Build history of the part. All positions in model axes, mm. Give positions to 0.01 mm unless a question says otherwise; leave off trailing zeros. Loops run counter-clockwise (first coordinate to the right, second up) from the corner with the lowest first, then second, coordinate; pieces in that order, holes last. Notation, with made-up numbers: (82.5, 31.25) -> (116.5, 31.25) arc R35 ccw to (116.5, 64.25) -> close; hole circle Ø3 at (46, 68). An arc over 180 degrees is marked (long way). Answer as a JSON object with one key per item and string values. Group by question number.
from build123d import *

# Parameters (mm, degrees)
SKETCH1_W           = 12.7
SKETCH1_H           = 20.32
BOSS_EXTRUDE1_DEPTH = 1
SKETCH2_R           = 0.5
SKETCH2_R_2         = 1.0922
CUT_EXTRUDE2_DEPTH  = 1
SKETCH3_W           = 0.7
SKETCH3_H           = 1.6
SKETCH3_W_2         = 2.149156966
SKETCH3_H_2         = 1.228089695
SKETCH3_W_3         = 4.14480272
SKETCH3_H_3         = 2.763201813
SKETCH3_W_4         = 0.8
SKETCH3_H_4         = 1.8
SKETCH3_W_5         = 1.6
SKETCH3_H_5         = 0.7
BOSS_EXTRUDE3_DEPTH = 0.75


with BuildPart() as part:
    # Sketch1 → Boss-Extrude1 (new body)
    with BuildSketch(Plane(origin=(0, 0, 0), x_dir=(1, 0, 0), z_dir=(0, 1, 0))):
        with Locations((6.35, 10.16)):
            Rectangle(SKETCH1_W, SKETCH1_H)
    extrude(amount=BOSS_EXTRUDE1_DEPTH)

    # Sketch2 → Cut-Extrude2 (cut)
    with BuildSketch(Plane(origin=(0, 1, 0), x_dir=(1, 0, 0), z_dir=(0, 1, 0))):
        with Locations(Location((1, 19.32, 0), (0, 0, 270))):
            Circle(SKETCH2_R)
        with Locations(Location((1, 16.702857143, 0), (0, 0, 270))):
            Circle(SKETCH2_R)
        with Locations(Location((1, 14.085714286, 0), (0, 0, 270))):
            Circle(SKETCH2_R)
        with Locations(Location((1, 11.468571429, 0), (0, 0, 270))):
            Circle(SKETCH2_R)
        with Locations(Location((1, 8.851428571, 0), (0, 0, 270))):
            Circle(SKETCH2_R)
        with Locations(Location((1, 6.234285714, 0), (0, 0, 270))):
            Circle(SKETCH2_R)
        with Locations(Location((1, 3.617142857, 0), (0, 0, 270))):
            Circle(SKETCH2_R)
        with Locations(Location((1, 1, 0), (0, 0, 270))):
            Circle(SKETCH2_R)
        with Locations(Location((10.7, 2, 0), (0, 0, 270))):
            Circle(SKETCH2_R_2)
    extrude(amount=-CUT_EXTRUDE2_DEPTH, mode=Mode.SUBTRACT)

    # Sketch3 → Boss-Extrude3 (add)
    with BuildSketch(Plane(origin=(0, 1, 0), x_dir=(1, 0, 0), z_dir=(0, 1, 0))):
        with Locations((9.600163685, 18.251782562)):
            Rectangle(SKETCH3_W, SKETCH3_H)
        with Locations((4.072917024, 18.06582741)):
            Rectangle(SKETCH3_W_2, SKETCH3_H_2)
        with Locations((8.908520197, 9.929733183)):
            Rectangle(SKETCH3_W_3, SKETCH3_H_3)
        with Locations((4.882280256, 4.84279592)):
            Rectangle(SKETCH3_W_4, SKETCH3_H_4)
        with Locations((4.472917024, 2.130764511)):
            Rectangle(SKETCH3_W_4, SKETCH3_H_4)
        with Locations((7.800163685, 18.251782562)):
            Rectangle(SKETCH3_W, SKETCH3_H)
        with Locations((11.400163685, 18.251782562)):
            Rectangle(SKETCH3_W, SKETCH3_H)
        with Locations((11.791455193, 14.963159232)):
            Rectangle(SKETCH3_W, SKETCH3_H)
        with Locations((3.286634502, 14.952625597)):
            Rectangle(SKETCH3_W_5, SKETCH3_H_5)
        with Locations((3.286634502, 13.813159232)):
            Rectangle(SKETCH3_W_5, SKETCH3_H_5)
        with Locations((8.005018674, 15.176499715)):
            Rectangle(SKETCH3_W_5, SKETCH3_H_5)
        with Locations((7.636118837, 13.813159232)):
            Rectangle(SKETCH3_W_5, SKETCH3_H_5)
        with Locations((3.808428935, 10.112643834)):
            Rectangle(SKETCH3_W, SKETCH3_H)
        with Locations((7.800163685, 5.771046806)):
            Rectangle(SKETCH3_W, SKETCH3_H)
        with Locations((9.155018674, 5.771046806)):
            Rectangle(SKETCH3_W, SKETCH3_H)
        with Locations((3.798338541, 7.466211291)):
            Rectangle(SKETCH3_W_5, SKETCH3_H_5)
    extrude(amount=BOSS_EXTRUDE3_DEPTH)


solid = part.part
(1) Saw through at A-A on x = 10.7. List the corners of the cut face in (y, z).
(2) Pull direction X, two halves, no side cores. Call faces 1 (the cylindrical face through (0.808, 0.507, -3.155)), 2 (the flat face through (9, 1.75, -10)), 3 (the flat face through (12.7, 0.5, -10)): pulls with the +X half, pulls with the -X half, needs draft (parallel to the pull), parting line crosses it, or undercut.
(3) Saw through at B-B on y = 0.4. Give the number of separate pieces and of enclosed holes in the cut face, plus the area to 3 significant figures.
(4) Pin check, flat tips, straight feed: pin 1 (0.8 mm diameter, centred on x = 3.5, y = 1.5, fed in from +Z); pin 2 (0.6 mm diameter, centred on x = 9, y = 1.5, fed in from +Z); pin 3 (0.6 mm diameter, centred on y = 1.5, z = -14.5, fed in from -X). Stop position of each tip, or through.
(5) Saw through at C-C on z = -19.32. List the corners of the cut face in (x, y).
(6) Probe line 1 along Z through (x, y) = (3.5, 1.65); line 2 along X through (y, z) = (1.35, -19); line 3 along X through (y, z) = (0.15, -11.5). List the from-to ranges inside material, lowest first. Write a range as [from, to].
(7) Saw through at D-D on x = 7.75. List the corners of the cut face in (y, z), plus the area to 3 significant figures.
Calculated:
{
 "1": {"outline": "(0, -20.32) -> (1, -20.32) -> (1, -11.31) -> (1.75, -11.31) -> (1.75, -8.55) -> (1, -8.55) -> (1, -3.09) -> (0, -3.09) -> close; (0, -0.91) -> (1, -0.91) -> (1, 0) -> (0, 0) -> close"},
 "2": {"face 1": "undercut", "face 2": "needs draft", "face 3": "pulls with the +X half"},
 "3": {"separate pieces": "1", "enclosed holes": "9", "area": "248 mm^2"},
 "4": {"pin 1": "stops at z = -7.12", "pin 2": "stops at z = -4.97", "pin 3": "stops at x = 2.49"},
 "5": {"outline": "(0, 0) -> (0.5, 0) -> (0.5, 1) -> (0, 1) -> close; (1.5, 0) -> (12.7, 0) -> (12.7, 1) -> (1.5, 1) -> close"},
 "6": {"line 1": "z = [-18.68, -17.45], [-15.3, -14.6], [-14.16, -13.46], [-10.91, -9.31], [-7.82, -7.12]", "line 2": "x = [7.45, 8.15], [9.25, 9.95], [11.05, 11.75]", "line 3": "x = [0, 0.5], [1.5, 12.7]"},
 "7": {"outline": "(0, -20.32) -> (1, -20.32) -> (1, -19.05) -> (1.75, -19.05) -> (1.75, -17.45) -> (1, -17.45) -> (1, -15.53) -> (1.75, -15.53) -> (1.75, -14.83) -> (1, -14.83) -> (1, -14.16) -> (1.75, -14.16) -> (1.75, -13.46) -> (1, -13.46) -> (1, -11.31) -> (1.75, -11.31) -> (1.75, -8.55) -> (1, -8.55) -> (1, -6.57) -> (1.75, -6.57) -> (1.75, -4.97) -> (1, -4.97) -> (1, 0) -> (0, 0) -> close", "area": "25.8 mm^2"}
}
